For this review, take the finished solid that the model builds, in its own axes (mm). A direction names the side the tool comes from. Round coordinates to 2 decimals unless told otherwise and drop trailing zeros. Order: outer loops, then holes, each group sorted by start corner. A loop starts at its lowest first (then second) coordinate and runs counter-clockwise, first axis right, second up. Notation, with made-up numbers: (67.5, 14.25) - (125.5, 14.25) arc R28 cw to (125.5, 52.25) - close; hole circle Ø2 at (14.25, 7.25). An arc over 180 degrees is marked (long way). One line per item, written item: value.
```python
from build123d import *

# Parameters (mm, degrees)
ESBO_O1_W                     = 16
ESBO_O1_H                     = 40
RESSALTO_EXTRUS_O1_DEPTH      = 2
ESBO_O2_R                     = 1.75
CORTE_EXTRUS_O1_DEPTH         = 2
ESBO_O3_W                     = 4.656179748
ESBO_O3_H                     = 12
RESSALTO_EXTRUS_O2_DEPTH      = 6
ESBO_O4_W                     = 12
ESBO_O4_H                     = 5
RESSALTO_EXTRUS_O3_DEPTH      = 6
RESSALTO_EXTRUS_O4_DEPTH      = 9
RESSALTO_EXTRUS_O4_DEPTH_BACK = 1.2
ESBO_O6_W                     = 3.964999664
ESBO_O6_H                     = 0.972728158


with BuildPart() as part:
    # Esboço1 → Ressalto-extrusão1 (new body)
    with BuildSketch(Plane.XY):
        Rectangle(ESBO_O1_W, ESBO_O1_H)
    extrude(amount=RESSALTO_EXTRUS_O1_DEPTH)

    # Esboço2 → Corte-extrusão1 (cut)
    with BuildSketch(Plane.XY.offset(2)):
        with Locations((-5.5, 16.5)):
            Circle(ESBO_O2_R)
        with Locations((-5.5, -2.5)):
            Circle(ESBO_O2_R)
    extrude(amount=-CORTE_EXTRUS_O1_DEPTH, mode=Mode.SUBTRACT)

    # Esboço3 → Ressalto-extrusão2 (add)
    with BuildSketch(Plane.XY.offset(2)):
        with Locations((-5.571910126, 7.2)):
            Rectangle(ESBO_O3_W, ESBO_O3_H)
    extrude(amount=RESSALTO_EXTRUS_O2_DEPTH)

    # Esboço4 → Ressalto-extrusão3 (add)
    with BuildSketch(Plane.XY.offset(2)):
        with Locations((0, -16.5)):
            Rectangle(ESBO_O4_W, ESBO_O4_H)
    extrude(amount=RESSALTO_EXTRUS_O3_DEPTH)

    # Esboço6 → Ressalto-extrusão4 (add, two sides: drawn at the far end of the back side and taken through both)
    with BuildSketch(Plane(origin=(-4.396287548, 12.767746119, 0), x_dir=(0, 0, -1), z_dir=(0.32556815445715404, -0.9455185755993177, 0)).offset(-RESSALTO_EXTRUS_O4_DEPTH_BACK)):
        with Locations((-5, -6.243358943)):
            Rectangle(ESBO_O6_W, ESBO_O6_H)
    extrude(amount=RESSALTO_EXTRUS_O4_DEPTH + RESSALTO_EXTRUS_O4_DEPTH_BACK)


solid = part.part
```
Item 1: Take a section at B-B (x = -5.5). Write out the cut boundary in (y, z).
Returned:
outline: (-20, 0) - (-4.25, 0) - (-4.25, 2) - (-14, 2) - (-14, 8) - (-19, 8) - (-19, 2) - (-20, 2) - close; (-0.75, 0) - (14.75, 0) - (14.75, 2) - (13.2, 2) - (13.2, 8) - (1.2, 8) - (1.2, 2) - (-0.75, 2) - close; (18.25, 0) - (20, 0) - (20, 2) - (18.25, 2) - close
Item 2: Take a section at D-D (x = -0.25). Write out the cut boundary in (y, z), plus the area to 3 significant figures.
Returned:
outline: (-20, 0) - (20, 0) - (20, 2) - (-14, 2) - (-14, 8) - (-19, 8) - (-19, 2) - (-20, 2) - close
area: 110 mm^2
Item 3: For P1, Ø8, axis at x = -4.5, y = -6, coming from the +Z side; P2, Ø10, axis at x = -2.5, y = 2, coming from the -Z side; P3, Ø1.6, axis at y = -7.5, z = 1, coming from the -X side; P4, Ø3.5, axis at x = -5, z = 5, coming from the -Y side, all flat-tipped, find the tip position at first contact; note any pin that passes through.
Returned:
P1: z = 2
P2: z = 0
P3: x = -8
P4: y = -19
Item 4: Take a section at A-A (z = 7.5). Write out the cut boundary in (x, y), plus the area to 3 significant figures.
Returned:
outline: (-7.9, 1.2) - (-3.24, 1.2) - (-3.24, 13.2) - (-7.9, 13.2) - close; (-6, -19) - (6, -19) - (6, -14) - (-6, -14) - close
area: 116 mm^2
Item 5: Wall thickness on line 1 (Y direction, x = -5.5, z = 1.4); line 2 (Y direction, x = -5.25, z = 3.5); line 3 (Z direction, x = -3.25, y = -10.5): over which ranges is each line inside the solid? List them lowest first.
Returned:
line 1: -20 to -4.25, -0.75 to 14.75, 18.25 to 20
line 2: -19 to -14, 1.2 to 13.2
line 3: 0 to 2
Item 6: Machinability: for faces 4 (the flat face through (6, -17, 5)), 5 (the flat face through (-9.5, 8.3, 6.982)), 6 (the flat face through (-6, 13.2, 5)), 7 (the flat face through (0, -14, 5)), 8 (the flat face through (0, -19, 5)), which of the approach directions +Z, -Z, +X, -X, +Y, -Y give a long, thin tool a straight path to every point of the face, cutting with its end or side? Answer none if there is none.
Returned:
face 4: +Z, +X, +Y, -Y
face 5: +Z, -X, +Y, -Y
face 6: +Z, +X, -X, +Y
face 7: +Z, +X, -X
face 8: +Z, +X, -X, -Y
Item 7: Take a section at C-C (y = 16.5). Write out the cut boundary in (x, z).
Returned:
outline: (-8, 0) - (-7.25, 0) - (-7.25, 2) - (-8, 2) - close; (-3.75, 0) - (8, 0) - (8, 2) - (-3.75, 2) - close
Item 8: The part is to be moulded in two halves that separate along X. For faces 1 (the flat face through (0, 0, 2)), 2 (the flat face through (-3.244, 7, 5)), 3 (the flat face through (-7.9, 7, 5)), say which applies: +X half, -X half, draft (parallel to the pull), parting line (faces both ways), or undercut.
Returned:
face 1: draft
face 2: +X half
face 3: undercut
